Geometry check sheet. Reference: drawing and pictorial views, mm from the part's lowest x, y, z. Coordinates: 2 decimals unless noted, no trailing zeros. Write each loop counter-clockwise with the first axis right and the second up, starting at its lowest first coordinate (ties: lowest second). Pieces come first, ordered by that corner, then holes. Notation, with made-up numbers: (43.5, 64.5) -> (76.5, 64.5) arc R18 cw to (76.5, 95.5) -> close; hole circle Ø9 at (-38.5, 66). An arc over 180 degrees is marked (long way). Use a Markdown table: item, result.
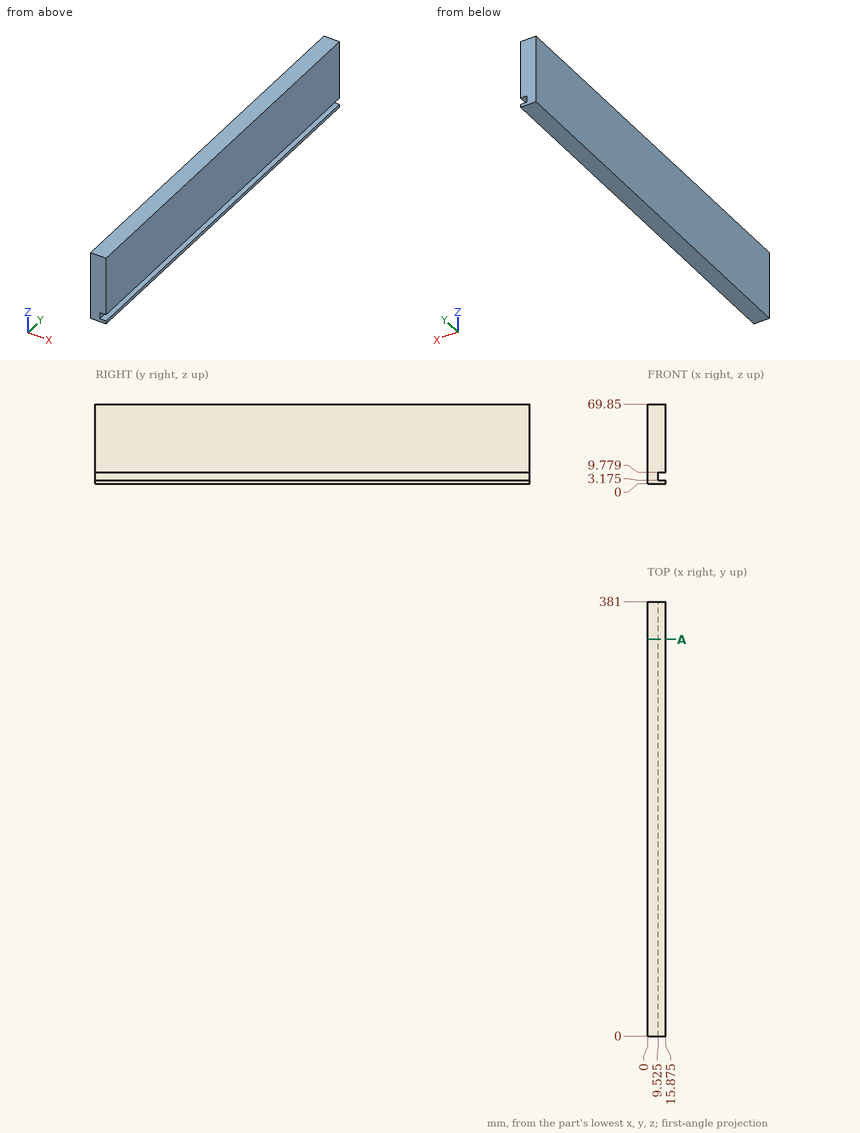
Item 1: Thickness scan on L1, parallel to Z at x = 11.25, y = 178 (3 decimals); L2, parallel to X at y = 134.5, z = 5 (3 decimals). Record the ranges inside material, lowest first. Write a range as [from, to].
Answer block:
| item | result |
|---|---|
| L1 | z = [0, 3.175], [9.779, 69.85] |
| L2 | x = [0, 9.525] |
Item 2: Section check A-A on y = 348. Record the boundary of the cut face in (x, z) (3 decimals), then the cut area to 3 significant figures.
Answer block:
| item | result |
|---|---|
| outline | (0, 0) -> (15.875, 0) -> (15.875, 3.175) -> (9.525, 3.175) -> (9.525, 9.779) -> (15.875, 9.779) -> (15.875, 69.85) -> (0, 69.85) -> close |
| area | 1,070 mm^2 |
Item 3: Depth check by flat-ended pin: P1, Ø4, axis at x = 6.5, z = 20.5, coming from the -Y side. Enter the tip coordinate at first touch or a pass-through.
Answer block:
| item | result |
|---|---|
| P1 | stops at y = 0 |
